Read the model definition and answer for the solid it produces. Units are mm, in the model's axes. Face numbers are marked on the shaded views. Give positions to 0.01 mm unless a question says otherwise; leave off trailing zeros. Loops run counter-clockwise (first coordinate to the right, second up) from the corner with the lowest first, then second, coordinate; pieces in that order, holes last.
(1) Find section D-D, the plane y = -4. State how many separate pieces and enclosed holes the cut face has, then the cut area to 3 significant figures.
(2) This flat-tipped pin is pushed along its axis until it touches: P1, Ø11, axis at x = -219, z = 50, coming from the +Y side. Where does it stop, or does it pass through?
(3) Determine the mould class of the marked faces 1 and 2 for opening direction Z: pulls with the +Z half, pulls with the -Z half, needs draft (parallel to the pull), parting line crosses it, or undercut.
(4) Find section C-C, the plane x = -163. Write down the section's boundary in (y, z).
(5) Find section B-B, the plane z = -50. Write down the section's boundary in (x, y), then the cut area to 3 significant figures.
(6) Straight lines are drawn through the part: probe 1 along X at (y, z) = (-3, -50); probe 2 along X at (y, z) = (-13.75, -16.5); probe 3 along Z at (x, y) = (-80, -14.5). For each, find the intervals that lie inside material, in ascending order.
(7) Find section A-A, the plane x = -114.5. Write down the section's boundary in (y, z), then the cut area to 3 significant figures.
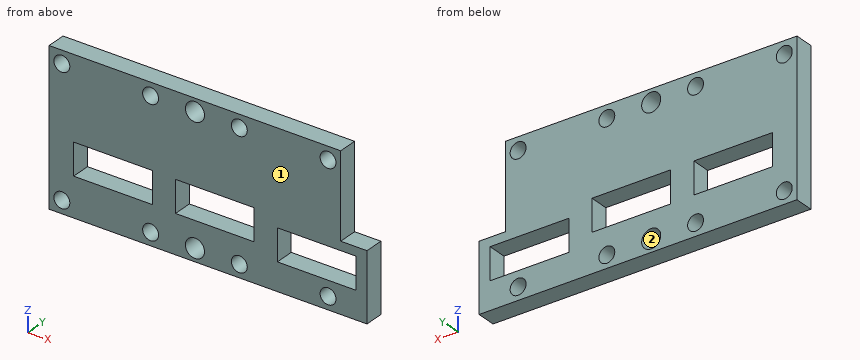
```python
from build123d import *

# Parameters (mm, degrees)
SKETCH1_W           = 229
SKETCH1_H           = 120
BOSS_EXTRUDE1_DEPTH = 15
SKETCH2_W           = 20.632503002
SKETCH2_H           = 53.730004003
BOSS_EXTRUDE2_DEPTH = 15
CUT_EXTRUDE1_REACH  = 239.205
SKETCH3_W           = 61.75
SKETCH3_H           = 25
CUT_EXTRUDE2_REACH  = 239.205
SKETCH4_W           = 61.75
SKETCH4_H           = 25
CUT_EXTRUDE3_REACH  = 239.205
SKETCH5_W           = 61.75
SKETCH5_H           = 25
CUT_EXTRUDE5_REACH  = 239.205
SKETCH7_R           = 7.5
CUT_EXTRUDE7_REACH  = 239.205
SKETCH14_R          = 6.25


with BuildPart() as part:
    # Sketch1 → Boss-Extrude1 (new body)
    with BuildSketch(Plane(origin=(0, 0, 0), x_dir=(1, 0, 0), z_dir=(0, 1, 0))):
        with Locations((-114.5, 0)):
            Rectangle(SKETCH1_W, SKETCH1_H)
    extrude(amount=-BOSS_EXTRUDE1_DEPTH)

    # Sketch2 → Boss-Extrude2 (add)
    with BuildSketch(Plane(origin=(0, 0, 0), x_dir=(1, 0, 0), z_dir=(0, 1, 0))):
        with Locations((10.316251501, 33.134997999)):
            Rectangle(SKETCH2_W, SKETCH2_H)
    extrude(amount=-BOSS_EXTRUDE2_DEPTH)

    # Sketch3 → Cut-Extrude1 (cut, up to next)
    with BuildSketch(Plane(origin=(0, 0, 0), x_dir=(1, 0, 0), z_dir=(0, 1, 0)), mode=Mode.PRIVATE) as cut_extrude1_sk1:
        with Locations((-18.875, 25.691000385)):
            Rectangle(SKETCH3_W, SKETCH3_H)
    cut_extrude1_tool1 = extrude(cut_extrude1_sk1.sketch, amount=-CUT_EXTRUDE1_REACH, mode=Mode.PRIVATE) & part.part
    add(cut_extrude1_tool1.solids().sort_by_distance((-18.875, 0, -25.691))[0], mode=Mode.SUBTRACT)

    # Sketch4 → Cut-Extrude2 (cut, up to next)
    with BuildSketch(Plane(origin=(0, 0, 0), x_dir=(1, 0, 0), z_dir=(0, 1, 0)), mode=Mode.PRIVATE) as cut_extrude2_sk1:
        with Locations((-98.875, 17.152366083)):
            Rectangle(SKETCH4_W, SKETCH4_H)
    cut_extrude2_tool1 = extrude(cut_extrude2_sk1.sketch, amount=-CUT_EXTRUDE2_REACH, mode=Mode.PRIVATE) & part.part
    add(cut_extrude2_tool1.solids().sort_by_distance((-98.875, 0, -17.152366))[0], mode=Mode.SUBTRACT)

    # Sketch5 → Cut-Extrude3 (cut, up to next)
    with BuildSketch(Plane(origin=(0, 0, 0), x_dir=(1, 0, 0), z_dir=(0, 1, 0)), mode=Mode.PRIVATE) as cut_extrude3_sk1:
        with Locations((-178.875, 16.78)):
            Rectangle(SKETCH5_W, SKETCH5_H)
    cut_extrude3_tool1 = extrude(cut_extrude3_sk1.sketch, amount=-CUT_EXTRUDE3_REACH, mode=Mode.PRIVATE) & part.part
    add(cut_extrude3_tool1.solids().sort_by_distance((-178.875, 0, -16.78))[0], mode=Mode.SUBTRACT)

    # Sketch7 → Cut-Extrude5 (cut, up to next)
    with BuildSketch(Plane(origin=(0, 0, 0), x_dir=(1, 0, 0), z_dir=(0, 1, 0)), mode=Mode.PRIVATE) as cut_extrude5_sk1:
        with Locations(Location((-114.5, 50, 0), (0, 0, 270))):
            Circle(SKETCH7_R)
    cut_extrude5_tool1 = extrude(cut_extrude5_sk1.sketch, amount=-CUT_EXTRUDE5_REACH, mode=Mode.PRIVATE) & part.part
    # Sketch7 → Cut-Extrude5 (cut, up to next)
    with BuildSketch(Plane(origin=(0, 0, 0), x_dir=(1, 0, 0), z_dir=(0, 1, 0)), mode=Mode.PRIVATE) as cut_extrude5_sk2:
        with Locations(Location((-114.5, -50, 0), (0, 0, 270))):
            Circle(SKETCH7_R)
    cut_extrude5_tool2 = extrude(cut_extrude5_sk2.sketch, amount=-CUT_EXTRUDE5_REACH, mode=Mode.PRIVATE) & part.part
    add(cut_extrude5_tool1.solids().sort_by_distance((-114.5, 0, -50))[0], mode=Mode.SUBTRACT)
    add(cut_extrude5_tool2.solids().sort_by_distance((-114.5, 0, 50))[0], mode=Mode.SUBTRACT)

    # Sketch14 → Cut-Extrude7 (cut, up to next)
    with BuildSketch(Plane(origin=(0, 0, 0), x_dir=(1, 0, 0), z_dir=(0, 1, 0)), mode=Mode.PRIVATE) as cut_extrude7_sk1:
        with Locations(Location((-219, 50, 0), (0, 0, 270))):
            Circle(SKETCH14_R)
    cut_extrude7_tool1 = extrude(cut_extrude7_sk1.sketch, amount=-CUT_EXTRUDE7_REACH, mode=Mode.PRIVATE) & part.part
    # Sketch14 → Cut-Extrude7 (cut, up to next)
    with BuildSketch(Plane(origin=(0, 0, 0), x_dir=(1, 0, 0), z_dir=(0, 1, 0)), mode=Mode.PRIVATE) as cut_extrude7_sk2:
        with Locations(Location((-219, -50, 0), (0, 0, 270))):
            Circle(SKETCH14_R)
    cut_extrude7_tool2 = extrude(cut_extrude7_sk2.sketch, amount=-CUT_EXTRUDE7_REACH, mode=Mode.PRIVATE) & part.part
    # Sketch14 → Cut-Extrude7 (cut, up to next)
    with BuildSketch(Plane(origin=(0, 0, 0), x_dir=(1, 0, 0), z_dir=(0, 1, 0)), mode=Mode.PRIVATE) as cut_extrude7_sk3:
        with Locations(Location((-149.323, -50, 0), (0, 0, 270))):
            Circle(SKETCH14_R)
    cut_extrude7_tool3 = extrude(cut_extrude7_sk3.sketch, amount=-CUT_EXTRUDE7_REACH, mode=Mode.PRIVATE) & part.part
    # Sketch14 → Cut-Extrude7 (cut, up to next)
    with BuildSketch(Plane(origin=(0, 0, 0), x_dir=(1, 0, 0), z_dir=(0, 1, 0)), mode=Mode.PRIVATE) as cut_extrude7_sk4:
        with Locations(Location((-79.646, -50, 0), (0, 0, 270))):
            Circle(SKETCH14_R)
    cut_extrude7_tool4 = extrude(cut_extrude7_sk4.sketch, amount=-CUT_EXTRUDE7_REACH, mode=Mode.PRIVATE) & part.part
    # Sketch14 → Cut-Extrude7 (cut, up to next)
    with BuildSketch(Plane(origin=(0, 0, 0), x_dir=(1, 0, 0), z_dir=(0, 1, 0)), mode=Mode.PRIVATE) as cut_extrude7_sk5:
        with Locations(Location((-9.969, -50, 0), (0, 0, 270))):
            Circle(SKETCH14_R)
    cut_extrude7_tool5 = extrude(cut_extrude7_sk5.sketch, amount=-CUT_EXTRUDE7_REACH, mode=Mode.PRIVATE) & part.part
    # Sketch14 → Cut-Extrude7 (cut, up to next)
    with BuildSketch(Plane(origin=(0, 0, 0), x_dir=(1, 0, 0), z_dir=(0, 1, 0)), mode=Mode.PRIVATE) as cut_extrude7_sk6:
        with Locations(Location((-9.969, 50, 0), (0, 0, 270))):
            Circle(SKETCH14_R)
    cut_extrude7_tool6 = extrude(cut_extrude7_sk6.sketch, amount=-CUT_EXTRUDE7_REACH, mode=Mode.PRIVATE) & part.part
    # Sketch14 → Cut-Extrude7 (cut, up to next)
    with BuildSketch(Plane(origin=(0, 0, 0), x_dir=(1, 0, 0), z_dir=(0, 1, 0)), mode=Mode.PRIVATE) as cut_extrude7_sk7:
        with Locations(Location((-79.646, 50, 0), (0, 0, 270))):
            Circle(SKETCH14_R)
    cut_extrude7_tool7 = extrude(cut_extrude7_sk7.sketch, amount=-CUT_EXTRUDE7_REACH, mode=Mode.PRIVATE) & part.part
    # Sketch14 → Cut-Extrude7 (cut, up to next)
    with BuildSketch(Plane(origin=(0, 0, 0), x_dir=(1, 0, 0), z_dir=(0, 1, 0)), mode=Mode.PRIVATE) as cut_extrude7_sk8:
        with Locations(Location((-149.323, 50, 0), (0, 0, 270))):
            Circle(SKETCH14_R)
    cut_extrude7_tool8 = extrude(cut_extrude7_sk8.sketch, amount=-CUT_EXTRUDE7_REACH, mode=Mode.PRIVATE) & part.part
    add(cut_extrude7_tool1.solids().sort_by_distance((-219, 0, -50))[0], mode=Mode.SUBTRACT)
    add(cut_extrude7_tool2.solids().sort_by_distance((-219, 0, 50))[0], mode=Mode.SUBTRACT)
    add(cut_extrude7_tool3.solids().sort_by_distance((-149.323, 0, 50))[0], mode=Mode.SUBTRACT)
    add(cut_extrude7_tool4.solids().sort_by_distance((-79.646, 0, 50))[0], mode=Mode.SUBTRACT)
    add(cut_extrude7_tool5.solids().sort_by_distance((-9.969, 0, 50))[0], mode=Mode.SUBTRACT)
    add(cut_extrude7_tool6.solids().sort_by_distance((-9.969, 0, -50))[0], mode=Mode.SUBTRACT)
    add(cut_extrude7_tool7.solids().sort_by_distance((-79.646, 0, -50))[0], mode=Mode.SUBTRACT)
    add(cut_extrude7_tool8.solids().sort_by_distance((-149.323, 0, -50))[0], mode=Mode.SUBTRACT)


solid = part.part
```
Entries:
1. separate pieces: 1
1. enclosed holes: 13
1. area: 22,600 mm2
2. P1: passes through
3. face 1: needs draft
3. face 2: undercut
4. outline: (-15, -60) - (0, -60) - (0, -29.28) - (-15, -29.28) - close; (-15, -4.28) - (0, -4.28) - (0, 60) - (-15, 60) - close
5. outline: (-229, -15) - (-225.25, -15) - (-225.25, 0) - (-229, 0) - close; (-212.75, -15) - (-155.57, -15) - (-155.57, 0) - (-212.75, 0) - close; (-143.07, -15) - (-122, -15) - (-122, 0) - (-143.07, 0) - close; (-107, -15) - (-85.9, -15) - (-85.9, 0) - (-107, 0) - close; (-73.4, -15) - (-16.22, -15) - (-16.22, 0) - (-73.4, 0) - close; (-3.72, -15) - (20.63, -15) - (20.63, 0) - (-3.72, 0) - close
5. area: 2,770 mm2
6. probe 1: x = -229 to -225.25, -212.75 to -155.57, -143.07 to -122, -107 to -85.9, -73.4 to -16.22, -3.72 to 20.63
6. probe 2: x = -229 to -209.75, -148 to -129.75, -68 to -49.75, 12 to 20.63
6. probe 3: z = -60 to -56.24, -43.76 to -29.65, -4.65 to 43.76, 56.24 to 60
7. outline: (-15, -60) - (0, -60) - (0, -57.5) - (-15, -57.5) - close; (-15, -42.5) - (0, -42.5) - (0, -29.65) - (-15, -29.65) - close; (-15, -4.65) - (0, -4.65) - (0, 42.5) - (-15, 42.5) - close; (-15, 57.5) - (0, 57.5) - (0, 60) - (-15, 60) - close
7. area: 975 mm2
